For this review, take the finished solid that the model builds, in its own axes (mm). A direction names the side the tool comes from. Round coordinates to 2 decimals unless told otherwise and drop trailing zeros. Write each loop counter-clockwise with the first axis right and the second up, starting at its lowest first coordinate (ties: lowest second). Pieces come first, ordered by that corner, then holes. Notation, with made-up numbers: (-19.5, -3.5) -> (6.5, -3.5) arc R13 ccw to (6.5, 12.5) -> close; hole circle Ø2 at (8, 50.25). An arc over 180 degrees is marked (long way). Answer in a Markdown table with one row per item.
Autodesk Inventor part; units mm, degrees
ref_plane "YZ Plane" through (0, 0, 0) normal (1, 0, 0) x (0, 1, 0)
ref_plane "XZ Plane" through (0, 0, 0) normal (0, 1, 0) x (-1, 0, 0)
ref_plane "XY Plane" through (0, 0, 0) normal (0, 0, 1) x (1, 0, 0)
sketch "Sketch1" plane through (0, 0, 0) normal (0, 0, 1) x (1, 0, 0)
  line L0 (8, -7.85) -> (-8, -7.85)
  line L1 (-8, 7.85) -> (8, 7.85)
  line L2 (8, -7.85) -> (-8, 7.85) construction
  line L3 (-9.5, -1.65) -> (-9.5, 1.65)
  line L4 (9.5, 1.65) -> (9.5, -1.65)
  line L5 (-8, -7.85) -> (-8, -1.65)
  line L6 (-8, 1.65) -> (-8, 7.85)
  line L7 (8, 7.85) -> (8, 1.65)
  line L8 (8, -1.65) -> (8, -7.85)
  line L9 (9.5, -1.65) -> (8, -1.65)
  line L10 (-8, -1.65) -> (-9.5, -1.65)
  line L11 (-9.5, 1.65) -> (-8, 1.65)
  line L12 (8, 1.65) -> (9.5, 1.65)
  point P0 (0, 0)
  dimension "d0" = 16
  dimension "d1" = 15.7
  dimension "d2" = 19
  dimension "d3" = 3.3
extrude "Extrusion1" add sketch "Sketch1" along normal blind 10
sketch "Sketch2" plane through (0, 0, 10) normal (0, 0, 1) x (1, 0, 0)
  circle A0 centre (0, 0) radius 7.05
  dimension "d6" = 14.1
extrude "Extrusion2" cut sketch "Sketch2" against normal blind 5
sketch "Sketch4" plane through (0, 0, 10) normal (0, 0, 1) x (1, 0, 0)
  circle A0 centre (0, 0) radius 8.75
  line L0 (-8, 1.65) -> (-8, 7.85)
  line L1 (0, 0) -> (-8, 7.85)
  line L2 (-8, -1.65) -> (-8, -7.85)
  line L3 (0, 0) -> (-8, -7.85)
  line L4 (-8, -7.85) -> (8, -7.85)
  line L5 (0, 0) -> (8, -7.85)
  line L6 (8, 7.85) -> (-8, 7.85)
  line L7 (0, 0) -> (8, 7.85)
  point P0 (-6.2455, 6.1284)
  point P1 (6.2455, 6.1284)
  point P2 (6.2455, -6.1284)
  point P3 (-6.2455, -6.1284)
  dimension "d17" = 17.5
hole "Hole2" at (-6.2455, 6.1284, 10) at (6.2455, 6.1284, 10) at (6.2455, -6.1284, 10) at (-6.2455, -6.1284, 10) direction (0, 0, -1) diameter 1.694 end through all
properties part number "teflonlense assem"
1) Mouldability with a two-part tool opening along X and no side actions: class faces 1 (the flat face through (9, 1.65, 5)), 2 (the cylindrical face through (6.208, 6.975, 4.93)), 3 (the flat face through (-8, 5, 5)) as pulls with the +X half, pulls with the -X half, needs draft (parallel to the pull), parting line crosses it, or undercut.
Solved:
| item | result |
|---|---|
| face 1 | needs draft |
| face 2 | undercut |
| face 3 | pulls with the -X half |
2) Consider section D-D on y = 0. State the section outline as (x, z) points.
Solved:
| item | result |
|---|---|
| outline | (-9.5, 0) -> (9.5, 0) -> (9.5, 10) -> (7.05, 10) -> (7.05, 5) -> (-7.05, 5) -> (-7.05, 10) -> (-9.5, 10) -> close |
3) Consider section C-C on z = 2.75. State the section outline as (x, y) points.
Solved:
| item | result |
|---|---|
| outline | (-9.5, -1.65) -> (-8, -1.65) -> (-8, -7.85) -> (8, -7.85) -> (8, -1.65) -> (9.5, -1.65) -> (9.5, 1.65) -> (8, 1.65) -> (8, 7.85) -> (-8, 7.85) -> (-8, 1.65) -> (-9.5, 1.65) -> close; hole circle Ø1.69 at (-6.25, -6.13); hole circle Ø1.69 at (-6.25, 6.13); hole circle Ø1.69 at (6.25, -6.13); hole circle Ø1.69 at (6.25, 6.13) |
4) For faces 4 (the flat face through (9, -1.65, 5)), 5 (the flat face through (0, 0, 5)), 6 (the flat face through (-9, -1.65, 5)), 7 (the flat face through (-9, 1.65, 5)), 8 (the cylindrical face through (-7.085, -6.018, 4.93)), list the 3-axis set-ups (+Z, -Z, +X, -X, +Y, -Y) from which the entire face can be reached by the end or side of a thin tool; tool diameter is ignored.
Solved:
| item | result |
|---|---|
| face 4 | +Z, -Z, +X, -Y |
| face 5 | +Z |
| face 6 | +Z, -Z, -X, -Y |
| face 7 | +Z, -Z, -X, +Y |
| face 8 | +Z, -Z |
5) For line 1 (Y direction, x = 0, z = 6.2); line 2 (Y direction, x = 5.75, z = 6); line 3 (X direction, y = -4.25, z = 2), list the stretches that pass through material, from the lowest coordinate up. Write a range as [from, to].
Solved:
| item | result |
|---|---|
| line 1 | [-7.85, -7.05], [7.05, 7.85] |
| line 2 | [-7.85, -6.82], [-5.44, -4.08], [4.08, 5.44], [6.82, 7.85] |
| line 3 | [-8, 8] |
6) Clearance check with flat-ended pins moving along their axes: pin 1 Ø3 at (y, z) = (5.5, 5) entering from +X; pin 2 Ø3 at (x, y) = (5, -0.5) entering from -Z; pin 3 Ø1 at (x, y) = (3, 2.5) entering from +Z; pin 4 Ø0.8 at (x, z) = (-8.5, 5) entering from -Y. State where each tip first meets the part, or that it passes through.
Solved:
| item | result |
|---|---|
| pin 1 | x = 8 |
| pin 2 | z = 0 |
| pin 3 | z = 5 |
| pin 4 | y = -1.65 |
7) Consider section A-A on x = 0. State the section outline as (y, z) points, then the cut area to 3 significant figures.
Solved:
| item | result |
|---|---|
| outline | (-7.85, 0) -> (7.85, 0) -> (7.85, 10) -> (7.05, 10) -> (7.05, 5) -> (-7.05, 5) -> (-7.05, 10) -> (-7.85, 10) -> close |
| area | 86.5 mm² |
8) Consider section B-B on y = -6.5. State the section outline as (x, z) points, then the cut area to 3 significant figures.
Solved:
| item | result |
|---|---|
| outline | (-8, 0) -> (-7.01, 0) -> (-7.01, 10) -> (-8, 10) -> close; (-5.48, 0) -> (5.48, 0) -> (5.48, 10) -> (2.73, 10) -> (2.73, 5) -> (-2.73, 5) -> (-2.73, 10) -> (-5.48, 10) -> close; (7.01, 0) -> (8, 0) -> (8, 10) -> (7.01, 10) -> close |
| area | 102 mm² |
